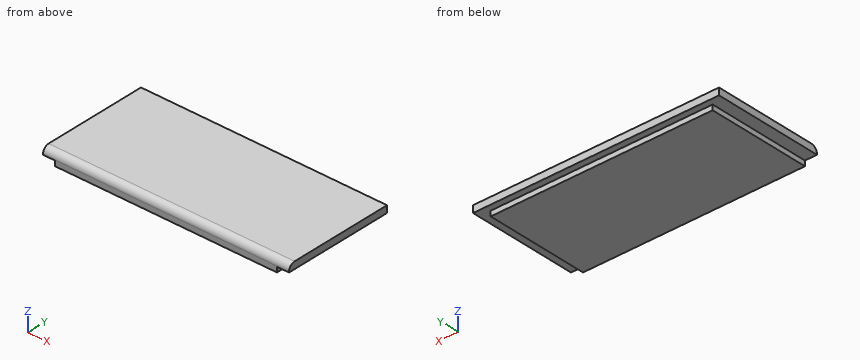
from build123d import *

# Parameters (mm, degrees)
F0_W     = 388
F0_H     = 174
F1_DEPTH = 19
F2_W     = 19
F2_H     = 8
F3_DEPTH = 178
F4_W     = 350
F4_H     = 8
F5_DEPTH = 10
F6_R     = 10


with BuildPart() as f1:
    # F0 (on Top) → F1 (new body)
    with BuildSketch(Plane.XY):
        Rectangle(F0_W, F0_H)
    extrude(amount=F1_DEPTH)

    # F2 (on face) → F3 (cut)
    with BuildSketch(Plane.XZ.offset(87)):
        with Locations((184.5, 4)):
            Rectangle(F2_W, F2_H)
        with Locations((-184.5, 4)):
            Rectangle(F2_W, F2_H)
    extrude(amount=-F3_DEPTH, mode=Mode.SUBTRACT)

    # F4 (on face) → F5 (cut)
    with BuildSketch(Plane(origin=(0, 87, 0), x_dir=(-1, 0, 0), z_dir=(0, 1, 0))):
        with Locations((0, 4)):
            Rectangle(F4_W, F4_H)
    extrude(amount=-F5_DEPTH, mode=Mode.SUBTRACT)

    # F6
    f6_edges = [f1.edges().sort_by_distance(p)[0] for p in [
        (0, -87, 19),
    ]]
    fillet(f6_edges, radius=F6_R)


solid = f1.part
Source: CAD feature listing. Evaluate the final solid. Frame: model axes, mm. Give positions to 0.01 mm unless a question says otherwise; leave off trailing zeros. Write each loop counter-clockwise with the first axis right and the second up, starting at its lowest first coordinate (ties: lowest second). Pieces come first, ordered by that corner, then holes. Notation, with made-up numbers: (-16, 56) -> (15, 56) arc R21 ccw to (15, 79) -> close; hole circle Ø7 at (75.5, 72). An arc over 180 degrees is marked (long way). Return JSON: item names as keys, results as strings. Group by question number.
1. Material intervals for line 1 (Y direction, x = 101, z = 7.5); line 2 (X direction, y = -21, z = 2.25); line 3 (Y direction, x = 129.5, z = 12), sorted ascending. Write a range as from..to.
2. Section C-C, the plane z = 3.5. Output: boundary loops of the cut face in (x, y).
3. Section A-A, the plane y = 28.5. Output: boundary loops of the cut face in (x, z).
4. Pin query (flat end, axial travel): pin 1 Ø1 at (x, z) = (107.5, 11) entering from -Y; pin 2 Ø6.5 at (x, z) = (38, 2) entering from +Y; pin 3 Ø9 at (y, z) = (21.5, 2.5) entering from +X. Return the tip coordinate at first contact, or that it passes through.
5. Section B-B, the plane x = -7.5. Output: boundary loops of the cut face in (y, z), then the cut area to 3 significant figures.
Determined:
{
 "1": {"line 1": "y = -87..77", "line 2": "x = -175..175", "line 3": "y = -86.54..87"},
 "2": {"outline": "(-175, -87) -> (175, -87) -> (175, 77) -> (-175, 77) -> close"},
 "3": {"outline": "(-194, 8) -> (-175, 8) -> (-175, 0) -> (175, 0) -> (175, 8) -> (194, 8) -> (194, 19) -> (-194, 19) -> close"},
 "4": {"pin 1": "stops at y = -86.89", "pin 2": "stops at y = 77", "pin 3": "stops at x = 175"},
 "5": {"outline": "(-87, 0) -> (77, 0) -> (77, 8) -> (87, 8) -> (87, 19) -> (-77, 19) arc R10 ccw to (-87, 9) -> close", "area": "3,200 mm2"}
}
